The listing builds one solid part. Answer for the finished solid, in the listing's coordinates (mm). A direction names the side the tool comes from. Round coordinates to 2 decimals unless told otherwise and drop trailing zeros. Loops run counter-clockwise (first coordinate to the right, second up) from the corner with the lowest first, then second, coordinate; pieces in that order, holes last. Notation, with made-up numbers: (87.25, 3.25) -> (133.25, 3.25) arc R25 cw to (133.25, 37.25) -> close; hole circle Ø1 at (87, 66). An arc over 180 degrees is marked (long way). Use a Markdown table: item, result. Add a question column.
Q1. Which of the six approach directions +Z, -Z, +X, -X, +Y, -Y give full straight-line access (tool end or side, diameter ignored) to faces 4 (the flat face through (12, -8, 7.2)), 5 (the flat face through (12, -13.696, 0)), 6 (the cylindrical face through (-97.25, -28.66, -5.4))?
Q2. Section B-B on x = -2 is taken. Give the vertices of the cut face in (y, z).
Q3. Given pin 1 Ø4.5 at (x, y) = (12.5, -9) entering from -Z; pin 2 Ø1 at (x, z) = (-24.5, -2.5) entering from +Y; pin 3 Ø3 at (x, z) = (13.5, 2) entering from +Y; pin 4 Ø4 at (x, y) = (-91.5, -27.5) entering from -Z, each flat-ended and moving along its own axis, determine where each tip first touches the part or whether it passes through.
Q4. Section A-A on z = 1.75 is taken. Give the vertices of the cut face in (x, y), then the cut area to 3 significant figures.
Q5. For a pull along Z with two mould halves and no side action, classify faces 1 (the flat face through (-55, -24, -10)), 2 (the flat face through (-92, -27, -6)), 3 (the flat face through (4.706, 1, 1)) as released by +Z, released by -Z, zero draft, split by the parting line, or undercut.
Q6. Consider line 1 (Z direction, x = 9, y = -8.5); line 2 (Y direction, x = -3, z = 3.5); line 3 (Z direction, x = -75, y = -34). Determine where each line is inside the solid, lowest interval first.
Autodesk Inventor part; units mm, degrees
ref_plane "Arbeitsebene2" through (4.7064, -12.4956, -10) normal (1, 0, 0) x (0, 0, -1)
ref_plane "YZ Plane" through (0, 0, 0) normal (1, 0, 0) x (0, 1, 0)
ref_plane "XZ Plane" through (0, 0, 0) normal (0, 1, 0) x (-1, 0, 0)
sketch "Skizze1" plane through (0, 0, 0) normal (0, 0, 1) x (1, 0, 0)
  line L0 (4.7064, 3.5044) -> (-12.7276, 3.5044)
  line L1 (-12.7276, 3.5044) -> (-116.0937, -34.1178)
  line L2 (4.7064, 3.5044) -> (4.7064, -16.4956)
  line L3 (4.7064, -16.4956) -> (-6.4216, -16.4956)
  line L4 (-6.4216, -16.4956) -> (-116.0937, -55.3341)
  line L5 (-116.0937, -34.1178) -> (-116.0937, -55.4014)
  line L6 (0, 15.2855) -> (0, -67.1826)
  line L7 (-140.2538, 0) -> (28.8665, 0)
  point P0 (0, 0)
  dimension "d0" = 17.434
  dimension "d1" = 110
  dimension "d4" = 20
  dimension "d5" = 11.128
  dimension "d38" = 4.7065
  dimension "d39" = 16.4956
  dimension "d40" = 20
  dimension "d44" = 160.499
ref_plane "Arbeitsebene2" through (4.7064, -12.4956, -10) normal (1, 0, 0) x (0, 0, -1)
sketch "Skizze3" plane through (4.7064, -12.4956, -10) normal (1, 0, 0) x (0, 0, -1)
  line L0 (-3, -65.9356) -> (-3, 0)
  line L1 (-17.2, 13.2) -> (-2.8, 13.2)
  line L2 (-2.8, 13.2) -> (-2.8, -1.2)
  line L3 (-2.8, -1.2) -> (-17.2, -1.2)
  line L4 (-17.2, -1.2) -> (-17.2, 13.2)
  line L5 (-4.8, 11.2) -> (-15.2, 11.2)
  line L6 (-15.2, 11.2) -> (-15.2, 0.8)
  line L7 (-15.2, 0.8) -> (-4.8, 0.8)
  line L8 (-4.8, 0.8) -> (-4.8, 11.2)
  line L9 (-2.8, -1.2) -> (-17.2, -1.2)
  line L10 (-17.2, -1.2) -> (-17.2, 13.2)
  point P0 (-3, -1.2)
  point P1 (-3, 0)
  dimension "d13" = 14.4
  dimension "d14" = 14.4
  dimension "d15" = 2
  dimension "d31" = 0
  dimension "d32" = 0
extrude "Extrusion2" add sketch "Skizze3" along normal blind 15 and the other way blind 7.5
sketch "Skizze5" plane through (-2.7936, -13.6956, 7.2) normal (0, 0, 1) x (1, 0, 0)
  circle A0 centre (13.5, 7.2) radius 1.6
  line L0 (22.5, 14.4) -> (22.5, 0)
  line L1 (0, 0) -> (22.5, 0)
  dimension "d29" = 3.2
  dimension "d47" = 7.2
  dimension "d48" = 9
extrude "Extrusion4" cut sketch "Skizze5" against normal up to surface (14.4 mm away)
extrude "Extrusion5" add sketch "Skizze1" along normal mid plane 20
shell "Wandung2" thickness 2.6 removed faces 2 at (-116.0937, -48.262, 3.3333) at (4.7064, -4.7623, 1.7333)
fillet "Rundung5" radius 4 8 edges at (-64.4106, -15.3067, 10) (-64.4106, -15.3067, -10) (-61.2576, -35.9149, 10) (-61.2576, -35.9149, -10) (-0.8576, -16.4956, 10) (-4.0106, 3.5044, 10) (-4.0106, 3.5044, -10) (-0.8576, -16.4956, -10)
sketch "Skizze6" plane through (-116.0937, -34.1178, 6) normal (-0.3420201, 0.9396926, 0) x (0.9396926, 0.3420201, 0)
  line L0 (31, 12) -> (19, 12)
  line L1 (19, 12) -> (19, 0)
  line L2 (19, 0) -> (31, 0)
  line L3 (31, 0) -> (31, 12)
  line L4 (109.2947, 16) -> (-1.4559, 16)
  line L5 (0, 0) -> (0, 12)
  point P0 (120.7614, 6)
  dimension "d49" = 12
  dimension "d50" = 12
  dimension "d51" = 4
  dimension "d52" = 19
extrude "Extrusion6" cut sketch "Skizze6" against normal blind 3
fillet "Rundung6" radius 2 4 edges at (-86.5186, -24.7368, -6) (-86.5186, -24.7368, 6) (-97.795, -28.8411, 6) (-97.795, -28.8411, -6)
sketch "Skizze7" plane through (0, 0, 10) normal (0, 0, 1) x (1, 0, 0)
  line L0 (-116.0937, -36.8847) -> (-116.0937, -52.5759)
  line L1 (-116.0937, -44.7303) -> (-90.1056, -35.2714)
  line L2 (-116.0937, -44.7303) -> (-88.4377, -44.7303) construction
  circle A0 centre (-108.0937, -41.8185) radius 1.6
  point P0 (0, 0)
  dimension "d56" = 20
  dimension "d57" = 3.2
  dimension "d58" = 8
extrude "Extrusion7" cut sketch "Skizze7" against normal up to surface (20 mm away)
sketch "Skizze8" plane through (0, 0, 0) normal (0, 0, 1) x (1, 0, 0)
  line L0 (68.2789, 41.5515) -> (-80.5987, 41.5515)
  line L1 (-80.5987, 41.5515) -> (-80.5987, -93.926)
  line L2 (-80.5987, -93.926) -> (68.2789, -93.926)
  line L3 (68.2789, -93.926) -> (68.2789, 41.5515)
  point P0 (0, 0)
properties part number "_3D-Druck"
Checked values:
| question | item | result |
|---|---|---|
| 1 | face 4 | +Z, +X, +Y, -Y |
| 1 | face 5 | +Z, -Z, +X, -Y |
| 1 | face 6 | +Y |
| 2 | outline | (-16.5, -6) arc R4 ccw to (-12.5, -10) -> (-0.5, -10) arc R4 ccw to (3.5, -6) -> (3.5, 6) arc R4 ccw to (-0.5, 10) -> (-12.5, 10) arc R4 ccw to (-16.5, 6) -> close; hole (-13.9, -7.4) -> (0.9, -7.4) -> (0.9, 7.4) -> (-13.9, 7.4) -> close |
| 3 | pin 1 | stops at z = -7.2 |
| 3 | pin 2 | stops at y = -0.6 |
| 3 | pin 3 | stops at y = 0.7 |
| 3 | pin 4 | stops at z = -10 |
| 4 | outline | (-116.09, -55.33) -> (-6.42, -16.5) -> (4.71, -16.5) -> (4.71, -13.7) -> (19.71, -13.7) -> (19.71, -11.7) -> (4.71, -11.7) -> (4.71, -11.1) -> (2.11, -11.1) -> (2.11, -13.9) -> (-6.87, -13.9) -> (-116.09, -52.58) -> close; (-116.09, -36.88) -> (-97.35, -30.06) -> (-98.24, -27.62) -> (-116.09, -34.12) -> close; (-86.96, -23.52) -> (-86.07, -25.96) -> (-12.27, 0.9) -> (2.11, 0.9) -> (2.11, -1.9) -> (4.71, -1.9) -> (4.71, -1.3) -> (19.71, -1.3) -> (19.71, 0.7) -> (4.71, 0.7) -> (4.71, 3.5) -> (-12.73, 3.5) -> close |
| 4 | area | 706 mm2 |
| 5 | face 1 | released by -Z |
| 5 | face 2 | undercut |
| 5 | face 3 | zero draft |
| 6 | line 1 | z = -7.2 to -5.2, 5.2 to 7.2 |
| 6 | line 2 | y = -16.5 to -13.9, 0.9 to 3.5 |
| 6 | line 3 | z = -10 to -7.4, 7.4 to 10 |
